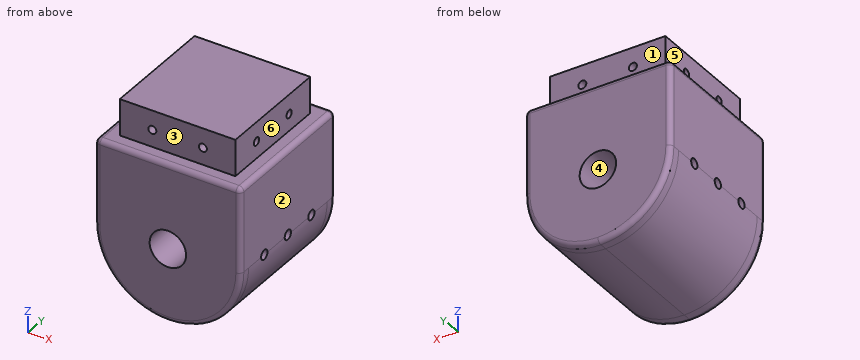
```python
from build123d import *

# Parameters (mm, degrees)
SKETCH2_W                  = 60
SKETCH2_H                  = 60
BOSS_EXTRUDE1_DEPTH        = 80
SKETCH3_OUTSIDE_W          = 85.324
SKETCH3_OUTSIDE_H          = 85.324
SKETCH3_OUTSIDE_W_2        = 47.6
SKETCH3_OUTSIDE_H_2        = 47.6
CUT_EXTRUDE1_DEPTH         = 15
SKETCH4_W                  = 60
SKETCH4_H                  = 5
CUT_EXTRUDE2_DEPTH         = 87
SKETCH5_R                  = 7.5
CUT_EXTRUDE3_DEPTH         = 87
M4_TAPPED_HOLE1_AT_2_COUNT = 2
M4_TAPPED_HOLE1_AT_2_PITCH = 20.8
CIRPATTERN1_COUNT          = 4
FILLET2_R                  = 30
SKETCH19_R                 = 2
CUT_EXTRUDE6_DEPTH         = 105.403065089
BOSS_EXTRUDE3_START        = 5
SKETCH21_R                 = 7.5
BOSS_EXTRUDE3_DEPTH        = 5
FILLET3_R                  = 2


with BuildPart() as part:
    # Sketch2 → Boss-Extrude1 (new body)
    with BuildSketch(Plane.XY):
        Rectangle(SKETCH2_W, SKETCH2_H)
    extrude(amount=BOSS_EXTRUDE1_DEPTH)

    # Sketch3 outside → Cut-Extrude1 (cut)
    with BuildSketch(Plane.XY.offset(80)):
        Rectangle(SKETCH3_OUTSIDE_W, SKETCH3_OUTSIDE_H)
        Rectangle(SKETCH3_OUTSIDE_W_2, SKETCH3_OUTSIDE_H_2, mode=Mode.SUBTRACT)
    extrude(amount=-CUT_EXTRUDE1_DEPTH, mode=Mode.SUBTRACT)

    # Sketch4 → Cut-Extrude2 (cut)
    with BuildSketch(Plane(origin=(30, 0, 0), x_dir=(0, 0, -1), z_dir=(1, 0, 0))):
        with Locations((-30, 27.5)):
            Rectangle(SKETCH4_W, SKETCH4_H)
        with Locations((-30, -27.5)):
            Rectangle(SKETCH4_W, SKETCH4_H)
    extrude(amount=-CUT_EXTRUDE2_DEPTH, mode=Mode.SUBTRACT)

    # Sketch5 → Cut-Extrude3 (cut)
    with BuildSketch(Plane(origin=(0, 25, 0), x_dir=(1, 0, 0), z_dir=(0, 1, 0))):
        with Locations(Location((0, -30, 0), (0, 0, 270))):
            Circle(SKETCH5_R)
    extrude(amount=-CUT_EXTRUDE3_DEPTH, mode=Mode.SUBTRACT)

    # Sketch16 → M4 Tapped Hole1 (revolve, cut)
    with BuildSketch(Plane(origin=(-23.8, 10.4, 72), x_dir=(0, 0, 1), z_dir=(0, 1, 0))):
        Polygon((0, 0), (0, 12.491420021), (1.65, 11.5), (1.65, 0), align=None)
    m4_tapped_hole1 = revolve(axis=Axis((-30.15, 10.4, 72), (1, 0, 0)), mode=Mode.SUBTRACT)

    # M4 Tapped Hole1 at 2: M4 Tapped Hole1 ×2
    with Locations(*[(0, -i * M4_TAPPED_HOLE1_AT_2_PITCH, 0) for i in range(1, M4_TAPPED_HOLE1_AT_2_COUNT)]):
        add(m4_tapped_hole1, mode=Mode.SUBTRACT)

    # CirPattern1: M4 Tapped Hole1 ×4 about axis
    cirpattern1_axis = Axis((0, 0, 0), (0, 0, 1))
    for i in range(1, CIRPATTERN1_COUNT):
        add(m4_tapped_hole1.rotate(cirpattern1_axis, i * 360 / CIRPATTERN1_COUNT), mode=Mode.SUBTRACT)

    # CirPattern1 copy 1 sketch → CirPattern1 copy 1 (revolve, cut)
    with BuildSketch(Plane(origin=(10.4, -23.8, 72), x_dir=(0, 0, 1), z_dir=(-1, 0, 0))):
        Polygon((0, 0), (0, 12.491420021), (1.65, 11.5), (1.65, 0), align=None)
    revolve(axis=Axis((10.4, -30.15, 72), (0, 1, 0)), mode=Mode.SUBTRACT)

    # CirPattern1 copy 2 sketch → CirPattern1 copy 2 (revolve, cut)
    with BuildSketch(Plane(origin=(23.8, 10.4, 72), x_dir=(0, 0, 1), z_dir=(0, -1, 0))):
        Polygon((0, 0), (0, 12.491420021), (1.65, 11.5), (1.65, 0), align=None)
    revolve(axis=Axis((30.15, 10.4, 72), (-1, 0, 0)), mode=Mode.SUBTRACT)

    # CirPattern1 copy 3 sketch → CirPattern1 copy 3 (revolve, cut)
    with BuildSketch(Plane(origin=(-10.4, 23.8, 72), x_dir=(0, 0, 1), z_dir=(1, 0, 0))):
        Polygon((0, 0), (0, 12.491420021), (1.65, 11.5), (1.65, 0), align=None)
    revolve(axis=Axis((-10.4, 30.15, 72), (0, -1, 0)), mode=Mode.SUBTRACT)

    # Fillet2
    fillet2_edges = [part.edges().sort_by_distance(p)[0] for p in [
        (30, 0, 0),
        (-30, 0, 0),
    ]]
    fillet(fillet2_edges, radius=FILLET2_R - 0.0001)  # a hair under: the kernel refuses the full size

    # Sketch19 → Cut-Extrude6 (cut, through all)
    with BuildSketch(Plane(origin=(30, 0, 0), x_dir=(0, 0, -1), z_dir=(1, 0, 0))):
        with Locations((-30, 0)):
            Circle(SKETCH19_R)
        with Locations((-30, 15)):
            Circle(SKETCH19_R)
        with Locations((-30, -15)):
            Circle(SKETCH19_R)
    extrude(amount=-CUT_EXTRUDE6_DEPTH, mode=Mode.SUBTRACT)

    # Sketch21 → Boss-Extrude3 (add)
    with BuildSketch(Plane(origin=(0, 25, 0), x_dir=(1, 0, 0), z_dir=(0, 1, 0)).offset(BOSS_EXTRUDE3_START)):
        with BuildLine():
            Line((30, -60), (30, -30))
            ThreePointArc((30, -30), (21.213203436, -8.786796564), (0, 0))
            ThreePointArc((0, 0), (-21.213203436, -8.786796564), (-30, -30))
            Line((-30, -30), (-30, -60))
            Line((-30, -60), (30, -60))
        make_face()
        with Locations(Location((0, -30, 0), (0, 0, 270))):
            Circle(SKETCH21_R, mode=Mode.SUBTRACT)
    boss_extrude3 = extrude(amount=-BOSS_EXTRUDE3_DEPTH)

    # Mirror4: Boss-Extrude3 across plane
    add(boss_extrude3.mirror(Plane.ZX))

    # Fillet3
    fillet3_edges = [part.edges().sort_by_distance(p)[0] for p in [
        (30, -30, 47.5),
        (-30, -30, 47.5),
        (0, -30, 65),
        (-30, 30, 47.5),
        (30, 30, 47.5),
        (0, 30, 0),
        (0, -30, 0),
        (30, 0, 65),
        (0, 30, 65),
        (-30, 0, 65),
    ]]
    fillet(fillet3_edges, radius=FILLET3_R)


solid = part.part
```
Work out the finished part from the listing and answer in its coordinate system (mm). Face numbers are marked on the shaded views. A direction names the side the tool comes from. Round coordinates to 2 decimals unless told otherwise and drop trailing zeros.
(1) For the marked faces 1 and 2, determine the directions among +Z, -Z, +X, -X, +Y, -Y from which every point of the face is accessible in a straight line to the end or side of a thin tool.
Computed values:
face 1: +Z, +X, -X, +Y
face 2: +Z, -Z, +X, +Y, -Y
(2) The part is cut by section A-A, the plane y = -15. Give the number of separate pieces and of enclosed holes in the cut face, and give its area (3 significant figures).
Computed values:
separate pieces: 2
enclosed holes: 2
area: 3,850 mm2
(3) Find the intervals of material crossed by L1, parallel to Y at x = 18, z = 72; L2, parallel to Y at x = -21, z = 30; L3, parallel to Z at x = 0.5, y = 0.5, in increasing order.
Computed values:
L1: y = -23.8 to -12.05, -8.75 to 8.75, 12.05 to 23.8
L2: y = -30 to -17, -13 to -2, 2 to 13, 17 to 30
L3: z = 0 to 22.52, 37.48 to 80
(4) The mould has two halves that part along X. Classify the marked faces 3, 4, 5 and 6: pulls with the +X half, pulls with the -X half, needs draft (parallel to the pull), parting line crosses it, or undercut.
Computed values:
face 3: needs draft
face 4: undercut
face 5: pulls with the -X half
face 6: pulls with the +X half
(5) Each of these flat-tipped pins is pushed along its axis until it touches: P1, Ø3, axis at y = 11, z = 70, coming from the -X side; P2, Ø3, axis at x = 10.4, z = 72, coming from the -Y side; P3, Ø19.5, axis at x = 0, z = 30, coming from the +Y side; P4, Ø1, axis at y = -16, z = 16.5, coming from the +X side. Where does it stop, or does it pass through?
Computed values:
P1: stops at x = -23.8
P2: stops at y = -12.21
P3: stops at y = 30
P4: stops at x = 27.04
